```python
from build123d import *

# Parameters (mm, degrees)
CROQUIS1_R              = 12.5
CROQUIS1_R_2            = 1.5
CROQUIS1_R_3            = 4
SALIENTE_EXTRUIR1_DEPTH = 1.2
CORTAR_EXTRUIR1_DEPTH   = 10
REDONDEO1_R             = 2


with BuildPart() as part:
    # Croquis1 → Saliente-Extruir1 (new body)
    with BuildSketch(Plane.XY):
        with Locations((-62.749306062, 7.483862191)):
            Circle(CROQUIS1_R)
        with Locations((-70.749306062, 7.483862191)):
            Circle(CROQUIS1_R_2, mode=Mode.SUBTRACT)
        with Locations((-54.749306062, 7.483862191)):
            Circle(CROQUIS1_R_2, mode=Mode.SUBTRACT)
        with Locations((-62.749306062, 16.983862191)):
            Circle(CROQUIS1_R_2, mode=Mode.SUBTRACT)
        with Locations((-62.749306062, -2.016137809)):
            Circle(CROQUIS1_R_2, mode=Mode.SUBTRACT)
        with Locations((-62.749306062, 7.483862191)):
            Circle(CROQUIS1_R_3, mode=Mode.SUBTRACT)
    extrude(amount=SALIENTE_EXTRUIR1_DEPTH)

    # Croquis2 → Cortar-Extruir1 (cut)
    with BuildSketch(Plane(origin=(0, 0, 0), x_dir=(-1, 0, 0), z_dir=(0, 0, -1))):
        with BuildLine():
            ThreePointArc((74.439306062, 11.910361937), (71.035706773, 16.842578089), (65.727627737, 19.623862191))
            ThreePointArc((65.727627737, 19.623862191), (68.485948691, 13.962864407), (74.439306062, 11.910361937))
        make_face()
        with BuildLine():
            ThreePointArc((74.439306062, 3.057362445), (71.035706773, -1.874853707), (65.727627737, -4.656137809))
            ThreePointArc((65.727627737, -4.656137809), (68.485948691, 1.004859975), (74.439306062, 3.057362445))
        make_face()
        with BuildLine():
            ThreePointArc((51.059306062, 3.057362445), (54.462905352, -1.874853707), (59.770984387, -4.656137809))
            ThreePointArc((59.770984387, -4.656137809), (57.012663434, 1.004859975), (51.059306062, 3.057362445))
        make_face()
        with BuildLine():
            ThreePointArc((51.059306062, 11.910361937), (54.462905352, 16.842578089), (59.770984387, 19.623862191))
            ThreePointArc((59.770984387, 19.623862191), (57.012663434, 13.962864407), (51.059306062, 11.910361937))
        make_face()
    extrude(amount=-CORTAR_EXTRUIR1_DEPTH, mode=Mode.SUBTRACT)

    # Redondeo1
    redondeo1_edges = [part.edges().sort_by_distance(p)[0] for p in [
        (-59.770984387, 19.623862191, 0.6),
        (-51.059306062, 11.910361937, 0.6),
        (-74.439306062, 11.910361937, 0.6),
        (-65.727627737, 19.623862191, 0.6),
        (-65.727627737, -4.656137809, 0.6),
        (-74.439306062, 3.057362445, 0.6),
        (-51.059306062, 3.057362445, 0.6),
        (-59.770984387, -4.656137809, 0.6),
    ]]
    fillet(redondeo1_edges, radius=REDONDEO1_R)


solid = part.part
```
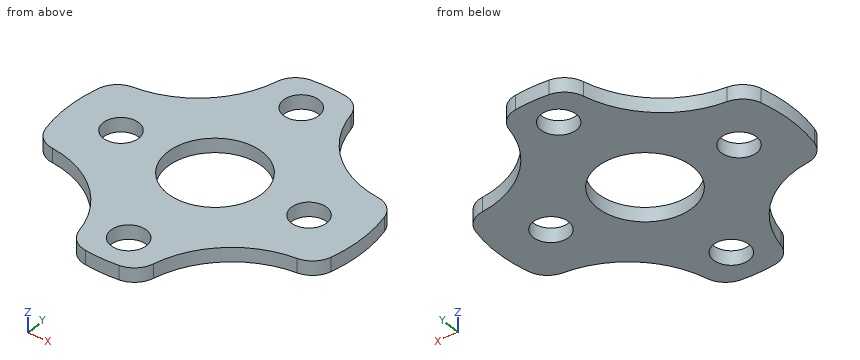
Check sheet for the modelled part. Datum: model origin and axes. Units: mm. Give positions to 0.01 mm unless a question says otherwise; leave off trailing zeros. Order: outer loops, then holes, each group sorted by start corner. A loop starts at its lowest first (then second) coordinate and runs counter-clockwise, first axis right, second up. Notation, with made-up numbers: (81, -16) -> (85, -16) arc R6 ccw to (85, -8) -> close; hole circle Ø1 at (1, -2.5). An arc over 180 degrees is marked (long way). Return JSON: item names as keys, results as strings.
1. Cross-section at C-C, the plane y = 6.5. Record the cut outline in (x, z).
From the geometry:
{"outline": "(-75.21, 0) -> (-71.88, 0) -> (-71.88, 1.2) -> (-75.21, 1.2) -> close; (-69.62, 0) -> (-66.63, 0) -> (-66.63, 1.2) -> (-69.62, 1.2) -> close; (-58.87, 0) -> (-55.88, 0) -> (-55.88, 1.2) -> (-58.87, 1.2) -> close; (-53.62, 0) -> (-50.29, 0) -> (-50.29, 1.2) -> (-53.62, 1.2) -> close"}
2. Cross-section at D-D, the plane x = -63. Record the cut outline in (y, z), plus the area to 3 significant figures.
From the geometry:
{"outline": "(-5.01, 0) -> (-3.5, 0) -> (-3.5, 1.2) -> (-5.01, 1.2) -> close; (-0.54, 0) -> (3.49, 0) -> (3.49, 1.2) -> (-0.54, 1.2) -> close; (11.48, 0) -> (15.5, 0) -> (15.5, 1.2) -> (11.48, 1.2) -> close; (18.46, 0) -> (19.98, 0) -> (19.98, 1.2) -> (18.46, 1.2) -> close", "area": "13.3 mm^2"}
3. Material ranges on probe 1 along X at (y, z) = (4.5, 1.1); probe 2 along Y at (x, z) = (-55.5, 0.5); probe 3 along Y at (x, z) = (-60.75, 1.05), recorded low to high. Write a range as [from, to].
From the geometry:
{"probe 1": "[-74.89, -65.41], [-60.09, -50.61]", "probe 2": "[2.07, 6.19], [8.78, 12.9]", "probe 3": "[-4.78, 4.02], [10.95, 19.75]"}
4. Cross-section at B-B, the plane x = -70.5. Record the cut outline in (y, z).
From the geometry:
{"outline": "(2.32, 0) -> (6, 0) -> (6, 1.2) -> (2.32, 1.2) -> close; (8.96, 0) -> (12.65, 0) -> (12.65, 1.2) -> (8.96, 1.2) -> close"}
5. Cross-section at A-A, the plane y = 10. Record the cut outline in (x, z).
From the geometry:
{"outline": "(-74.99, 0) -> (-65.86, 0) -> (-65.86, 1.2) -> (-74.99, 1.2) -> close; (-59.64, 0) -> (-50.51, 0) -> (-50.51, 1.2) -> (-59.64, 1.2) -> close"}
6. Go/stop test with a flat-tipped pin: P1, Ø7, axis at x = -62.75, y = 7.48, coming from the +Z side. Record where the tip stops, or that it passes through.
From the geometry:
{"P1": "through"}
